Build history of the part. All positions in model axes, mm. A direction names the side the tool comes from. Give positions to 0.01 mm unless a question says otherwise; leave off trailing zeros. Loops run counter-clockwise (first coordinate to the right, second up) from the corner with the lowest first, then second, coordinate; pieces in that order, holes last. Notation, with made-up numbers: (86, 18) -> (137, 18) arc R24 ccw to (137, 57) -> close; hole circle Ø11 at (-37.5, 86). An arc over 180 degrees is marked (long way). Answer as a JSON object with one key per item and string values. Group by question number.
Q1. Wall check: probe 1 along Y at (x, z) = (-1.6, 1.6); probe 2 along X at (y, z) = (21, -0.05); probe 3 along Y at (x, z) = (0.9, 0.1). Give the ranges that are in metal, low to high. Write a range as from..to.
Q2. Tool access for faces 1 (the flat face through (-1, 0, -1)), 2 (the flat face through (-1, -2, -1)): list every direction of +Z, -Z, +X, -X, +Y, -Y with a clear straight run to the whole face (end or side of a thin tool).
Q3. Band-saw the part on A-A, the plane z = 0. Write the cut outline in (x, y), plus the area to 3 significant figures.
Q4. Band-saw the part on D-D, the plane x = 1.25. Write the cut outline in (y, z).
Q5. Band-saw the part on C-C, the plane y = 6.5. Write the cut outline in (x, z), plus the area to 3 significant figures.
Q6. Two-plate mould, pull along X, no slides. Class faces 3 (the cylindrical face through (-2.44, -0.99, 0.54)), 4 (the flat face through (0, -1.5, 0)), 5 (the flat face through (0, 24, 0)): pulls with the +X half, pulls with the -X half, needs draft (parallel to the pull), parting line crosses it, or undercut.
Q7. Band-saw the part on B-B, the plane x = 0. Write the cut outline in (y, z).
Q8. Drop flat-ended pins along their axis: pin 1 (3 mm diameter, centred on y = 13.5, z = -1, fed in from -X); pin 2 (1 mm diameter, centred on x = -2, y = 17, fed in from +Z); pin 3 (2 mm diameter, centred on x = 0.5, y = 3.5, fed in from +Z). Give the stop position or say it passes through.
from build123d import *

# Parameters (mm, degrees)
SKETCH1_R           = 1
BOSS_EXTRUDE1_DEPTH = 24
SKETCH2_R           = 2.5
BOSS_EXTRUDE2_DEPTH = 2
SKETCH3_W           = 1.65
SKETCH3_H           = 1
SKETCH3_W_2         = 1
SKETCH3_H_2         = 1.65
CUT_EXTRUDE1_DEPTH  = 0.5
FILLET1_R           = 0.2


with BuildPart() as part:
    # Sketch1 → Boss-Extrude1 (new body)
    with BuildSketch(Plane(origin=(0, 0, 0), x_dir=(1, 0, 0), z_dir=(0, 1, 0))):
        with Locations(Location((0, 0, 0), (0, 0, 270))):
            Circle(SKETCH1_R)
    extrude(amount=BOSS_EXTRUDE1_DEPTH)

    # Sketch2 → Boss-Extrude2 (add)
    with BuildSketch(Plane.XZ):
        with Locations(Location((0, 0, 0), (0, 0, 270))):
            Circle(SKETCH2_R)
    extrude(amount=BOSS_EXTRUDE2_DEPTH)

    # Sketch3 → Cut-Extrude1 (cut)
    with BuildSketch(Plane.XZ.offset(2)):
        with Locations((1.325, 0)):
            Rectangle(SKETCH3_W, SKETCH3_H)
        with Locations((0, -1.325)):
            Rectangle(SKETCH3_W_2, SKETCH3_H_2)
        with Locations((-1.325, 0)):
            Rectangle(SKETCH3_W, SKETCH3_H)
        with Locations((0, 1.325)):
            Rectangle(SKETCH3_W_2, SKETCH3_H_2)
        Rectangle(SKETCH3_W_2, SKETCH3_H)
    extrude(amount=-CUT_EXTRUDE1_DEPTH, mode=Mode.SUBTRACT)

    # Fillet1
    fillet1_edges = [part.edges().sort_by_distance(p)[0] for p in [
        (1.325, -1.5, -0.5),
        (0.5, -1.5, -1.325),
        (0, -1.5, -2.15),
        (-1.325, -1.5, -0.5),
        (0.5, -1.5, 1.325),
        (2.15, -1.5, 0),
        (-0.5, -1.5, -1.325),
        (-2.15, -1.5, 0),
        (-1.325, -1.5, 0.5),
        (-0.5, -1.5, 1.325),
        (0, -1.5, 2.15),
        (1.325, -1.5, 0.5),
    ]]
    fillet(fillet1_edges, radius=FILLET1_R)


solid = part.part
Worked answers:
{
 "1": {"probe 1": "-2..0", "probe 2": "-1..1", "probe 3": "-1.5..24"},
 "2": {"face 1": "+Y", "face 2": "+Z, -Z, +X, -X, -Y"},
 "3": {"outline": "(-2.5, -2) -> (-2.15, -2) -> (-2.15, -1.7) arc R0.2 cw to (-1.95, -1.5) -> (1.95, -1.5) arc R0.2 cw to (2.15, -1.7) -> (2.15, -2) -> (2.5, -2) -> (2.5, 0) -> (1, 0) -> (1, 24) -> (-1, 24) -> (-1, 0) -> (-2.5, 0) -> close", "area": "55.9 mm2"},
 "4": {"outline": "(-2, -2.17) -> (0, -2.17) -> (0, 2.17) -> (-2, 2.17) -> (-2, 0.5) -> (-1.7, 0.5) arc R0.2 cw to (-1.5, 0.3) -> (-1.5, -0.3) arc R0.2 cw to (-1.7, -0.5) -> (-2, -0.5) -> close"},
 "5": {"outline": "circle Ø2 at (0, 0)", "area": "3.14 mm2"},
 "6": {"face 3": "parting line crosses it", "face 4": "undercut", "face 5": "needs draft"},
 "7": {"outline": "(-2, -2.5) -> (0, -2.5) -> (0, -1) -> (24, -1) -> (24, 1) -> (0, 1) -> (0, 2.5) -> (-2, 2.5) -> (-2, 2.15) -> (-1.7, 2.15) arc R0.2 cw to (-1.5, 1.95) -> (-1.5, -1.95) arc R0.2 cw to (-1.7, -2.15) -> (-2, -2.15) -> close"},
 "8": {"pin 1": "x = -1", "pin 2": "through", "pin 3": "z = 1"}
}
